Autodesk Inventor part; units mm, degrees
ref_plane "YZ Plane" through (0, 0, 0) normal (1, 0, 0) x (0, 1, 0)
ref_plane "XZ Plane" through (0, 0, 0) normal (0, 1, 0) x (-1, 0, 0)
ref_plane "XY Plane" through (0, 0, 0) normal (0, 0, 1) x (1, 0, 0)
sketch "Skizze1" plane through (0, 0, 0) normal (0, 1, 0) x (-1, 0, 0)
  circle A0 centre (0, 0) radius 1.85
  circle A1 centre (0, 0) radius 5
  line L0 (0, 0) -> (0, -12) construction
  arc A2 (5, -17) -> (-5, -17) centre (0, -17) ccw
  line L1 (5, 0) -> (5, -17)
  line L2 (-5, 0) -> (-5, -17)
  dimension "d0" = 3.7
  dimension "d1" = 10
extrude "Extrusion1" add sketch "Skizze1" along normal blind 1.8
properties part number "chain_elmt_1"
Read the model definition and answer for the solid it produces. Units are mm, in the model's axes. Give positions to 0.01 mm unless a question says otherwise; leave off trailing zeros. Order: outer loops, then holes, each group sorted by start corner. A loop starts at its lowest first (then second) coordinate and runs counter-clockwise, first axis right, second up. Notation, with made-up numbers: (57.5, -6.75) -> (67.5, -6.75) arc R31 cw to (67.5, 17.25) -> close; hole circle Ø10 at (63.5, 14). An arc over 180 degrees is marked (long way). One line per item, written item: value. Start each with the question number.
(1) Straight lines are drawn through the part: L1, parallel to Z at x = 0, y = 1.1; L2, parallel to X at y = 0.45, z = -12.5; L3, parallel to Z at x = 1, y = 1.3. For each, find the intervals that lie inside material, in ascending order.
(2) The part is cut by section B-B (x = 0). Determine the outline of the cut face in (y, z), and give its area (3 significant figures).
(3) For a pull along X with two mould halves and no side action, classify faces 1 (the flat face through (0, 1.8, -6)), 2 (the cylindrical face through (0, 1, -12)), 3 (the flat face through (5, 1, -8)) as released by +X, released by -X, zero draft, split by the parting line, or undercut.
(4) The part is cut by section C-C (y = 1.6). Determine the outline of the cut face in (x, z).
(5) The part is cut by section D-D (z = 3). Determine the outline of the cut face in (x, y).
(6) The part is cut by section A-A (z = -13). Determine the outline of the cut face in (x, y).
Taken from the geometry:
1. L1: -12 to -1.85, 1.85 to 5
1. L2: -5 to -2.18, 2.18 to 5
1. L3: -12.1 to -1.56, 1.56 to 4.9
2. outline: (0, -12) -> (1.8, -12) -> (1.8, -1.85) -> (0, -1.85) -> close; (0, 1.85) -> (1.8, 1.85) -> (1.8, 5) -> (0, 5) -> close
2. area: 23.9 mm^2
3. face 1: zero draft
3. face 2: undercut
3. face 3: released by +X
4. outline: (-5, -17) arc R5 cw to (5, -17) -> (5, 0) arc R5 ccw to (-5, 0) -> close; hole circle Ø3.7 at (0, 0)
5. outline: (-4, 0) -> (4, 0) -> (4, 1.8) -> (-4, 1.8) -> close
6. outline: (-5, 0) -> (-3, 0) -> (-3, 1.8) -> (-5, 1.8) -> close; (3, 0) -> (5, 0) -> (5, 1.8) -> (3, 1.8) -> close
